Check sheet for the modelled part. Datum: model origin and axes. Units: mm. Face numbers are marked on the shaded views. A direction names the side the tool comes from. Round coordinates to 2 decimals unless told otherwise and drop trailing zeros. Write each loop counter-clockwise with the first axis right and the second up, starting at its lowest first coordinate (ties: lowest second). Pieces come first, ordered by that corner, then holes.
Item 1: Release check for a two-part mould opening along Z. For the marked faces 1, 2 and 3 record: pulls with the +Z half, pulls with the -Z half, needs draft (parallel to the pull), parting line crosses it, or undercut.
Item 2: Material ranges on line 1 along X through (y, z) = (13.55, -44); line 2 along Z through (x, y) = (-25.5, 3.25); line 3 along X through (y, z) = (10.75, 29), recorded low to high.
Item 3: Section check D-D, the plane z = 23. Record the cut outline in (x, y), plus the area to 3 significant figures.
Item 4: Section check C-C, the plane x = 26. Record the cut outline in (y, z), plus the area to 3 significant figures.
Item 5: Depth check by flat-ended pin: pin 1 (3.5 mm diameter, centred on x = 34, z = -23, fed in from -Y); pin 2 (2.5 mm diameter, centred on x = 26, y = 8, fed in from +Z); pin 3 (5 mm diameter, centred on x = -36, z = -10, fed in from -Y). Enter the tip coordinate at first touch or a pass-through.
Item 6: Set-up check for the marked faces 4 and 5: record each of +Z, -Z, +X, -X, +Y, -Y from which the full face is reachable in a straight line by a thin tool's end or side.
Item 7: Section check B-B, the plane y = 8. Record the cut outline in (x, z).
Item 8: Section check A-A, the plane z = 0.5. Record the cut outline in (x, y), plus the area to 3 significant figures.
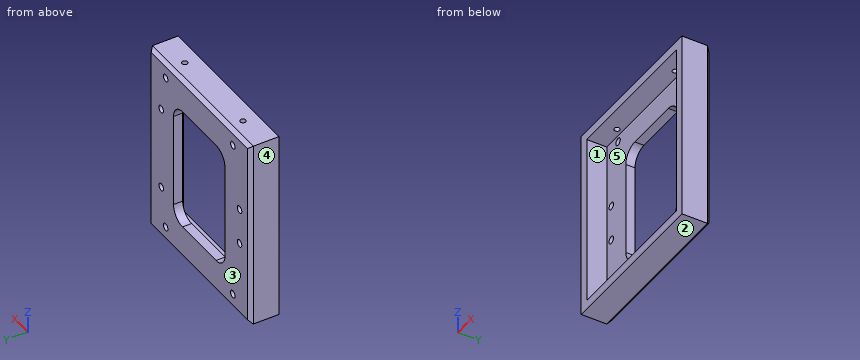
from build123d import *

# Parameters (mm, degrees)
SKETCH1_W           = 90
SKETCH1_H           = 105
BOSS_EXTRUDE1_DEPTH = 16
CHAMFER1_SIZE       = 2
SKETCH3_W           = 80
SKETCH3_H           = 95
CUT_EXTRUDE1_DEPTH  = 11
CUT_EXTRUDE2_DEPTH  = 71.973586636
SKETCH5_R           = 2
CUT_EXTRUDE3_DEPTH  = 71.973586636
SKETCH6_R           = 1.5
CUT_EXTRUDE4_DEPTH  = 5


with BuildPart() as part:
    # Sketch1 → Boss-Extrude1 (new body)
    with BuildSketch(Plane(origin=(0, 0, 0), x_dir=(1, 0, 0), z_dir=(0, 1, 0))):
        Rectangle(SKETCH1_W, SKETCH1_H)
    extrude(amount=BOSS_EXTRUDE1_DEPTH)

    # Chamfer1
    chamfer1_edges = [part.edges().sort_by_distance(p)[0] for p in [
        (-45, 16, 0),
        (0, 16, 52.5),
        (45, 16, 0),
        (0, 16, -52.5),
    ]]
    chamfer(chamfer1_edges, length=CHAMFER1_SIZE)

    # Sketch3 → Cut-Extrude1 (cut)
    with BuildSketch(Plane.XZ):
        Rectangle(SKETCH3_W, SKETCH3_H)
    extrude(amount=-CUT_EXTRUDE1_DEPTH, mode=Mode.SUBTRACT)

    # Sketch4 → Cut-Extrude2 (cut, through all)
    with BuildSketch(Plane(origin=(0, 16, 0), x_dir=(1, 0, 0), z_dir=(0, 1, 0))):
        with BuildLine():
            Line((-15, 34), (15, 34))
            ThreePointArc((15, 34), (20.656854249, 31.656854249), (23, 26))
            Line((23, 26), (23, -26))
            ThreePointArc((23, -26), (20.656854249, -31.656854249), (15, -34))
            Line((15, -34), (-15, -34))
            ThreePointArc((-15, -34), (-20.656854249, -31.656854249), (-23, -26))
            Line((-23, -26), (-23, 26))
            ThreePointArc((-23, 26), (-20.656854249, 31.656854249), (-15, 34))
        make_face()
    extrude(amount=-CUT_EXTRUDE2_DEPTH, mode=Mode.SUBTRACT)

    # Sketch5 → Cut-Extrude3 (cut, through all)
    with BuildSketch(Plane(origin=(0, 16, 0), x_dir=(1, 0, 0), z_dir=(0, 1, 0))):
        with Locations(Location((-30, 44, 0), (0, 0, 270))):
            Circle(SKETCH5_R)
        with Locations(Location((-30, -44, 0), (0, 0, 270))):
            Circle(SKETCH5_R)
        with Locations(Location((30, -44, 0), (0, 0, 270))):
            Circle(SKETCH5_R)
        with Locations(Location((30, 44, 0), (0, 0, 270))):
            Circle(SKETCH5_R)
        with Locations(Location((-36, -10, 0), (0, 0, 270))):
            Circle(SKETCH5_R)
        with Locations(Location((34, 23, 0), (0, 0, 270))):
            Circle(SKETCH5_R)
        with Locations(Location((-36, 10, 0), (0, 0, 270))):
            Circle(SKETCH5_R)
        with Locations(Location((34, -23, 0), (0, 0, 270))):
            Circle(SKETCH5_R)
    extrude(amount=-CUT_EXTRUDE3_DEPTH, mode=Mode.SUBTRACT)

    # Sketch6 → Cut-Extrude4 (cut)
    with BuildSketch(Plane.XY.offset(52.5)):
        with Locations((-26, 8)):
            Circle(SKETCH6_R)
        with Locations((26, 8)):
            Circle(SKETCH6_R)
    extrude(amount=-CUT_EXTRUDE4_DEPTH, mode=Mode.SUBTRACT)


solid = part.part
Values found:
1. face 1: undercut
1. face 2: pulls with the -Z half
1. face 3: needs draft
2. line 1: x = -45 to -32, -28 to 28, 32 to 45
2. line 2: z = -52.5 to -47.5, 47.5 to 52.5
2. line 3: x = -45 to -40, 40 to 45
3. outline: (-45, 0) - (-40, 0) - (-40, 11) - (-23, 11) - (-23, 16) - (-43, 16) - (-45, 14) - close; (23, 11) - (32, 11) - (32, 16) - (23, 16) - close; (36, 11) - (40, 11) - (40, 0) - (45, 0) - (45, 14) - (43, 16) - (36, 16) - close
3. area: 306 mm2
4. outline: (0, -52.5) - (14, -52.5) - (16, -50.5) - (16, 50.5) - (14, 52.5) - (9.5, 52.5) - (9.5, 47.5) - (11, 47.5) - (11, -47.5) - (0, -47.5) - close; (0, 47.5) - (6.5, 47.5) - (6.5, 52.5) - (0, 52.5) - close
4. area: 616 mm2
5. pin 1: passes through
5. pin 2: stops at z = -47.5
5. pin 3: stops at y = 11
6. face 4: +Z, -Z, -X, +Y, -Y
6. face 5: -Y
7. outline: (-45, -52.5) - (45, -52.5) - (45, 52.5) - (27.5, 52.5) - (27.5, 47.5) - (40, 47.5) - (40, -47.5) - (-40, -47.5) - (-40, 47.5) - (-27.5, 47.5) - (-27.5, 52.5) - (-45, 52.5) - close; (-24.5, 47.5) - (24.5, 47.5) - (24.5, 52.5) - (-24.5, 52.5) - close
8. outline: (-45, 0) - (-40, 0) - (-40, 11) - (-23, 11) - (-23, 16) - (-43, 16) - (-45, 14) - close; (23, 11) - (40, 11) - (40, 0) - (45, 0) - (45, 14) - (43, 16) - (23, 16) - close
8. area: 326 mm2
